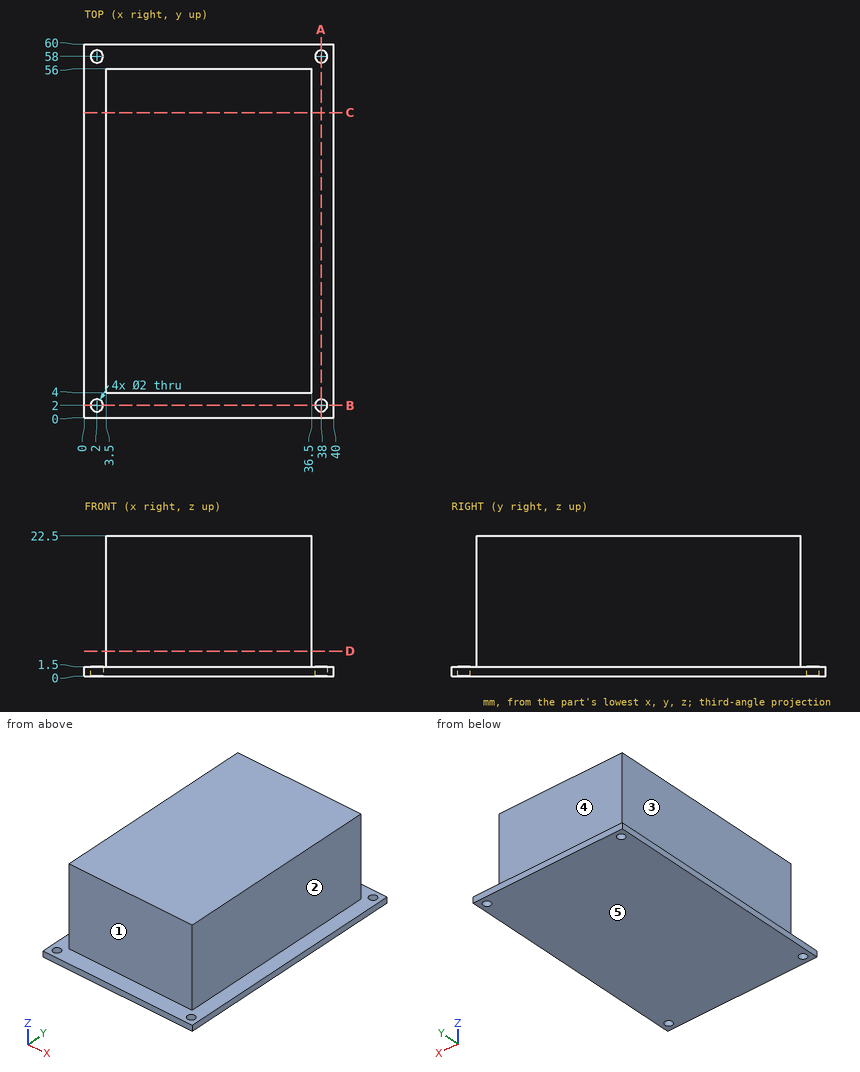
Job drawing, mm, ordinate dimensions from the low corner. One solid piece. A direction names the side the tool comes from. Give positions to 0.01 mm unless a question says otherwise; leave off trailing zeros. Loops run counter-clockwise (first coordinate to the right, second up) from the corner with the lowest first, then second, coordinate; pieces in that order, holes last. Notation, with made-up numbers: M 60,82.5 L 100,82.5 A19 cw 100,112.5 Z; hole C 66.5,44 d6. An arc over 180 degrees is marked long. Put each result on its own line as item: value. Start each with the question number.
1) 3-axis set-ups, long thin cutter, end or side, ignore diameter. For the marked faces 4 and 5: which of +Z, -Z, +X, -X, +Y, -Y reach the whole face in a straight line?
2) Flat gauge pins, fed straight in: pin 1 (6.5 mm diameter, centred on x = 19.5, z = 8, fed in from +Y); pin 2 (1.5 mm diameter, centred on x = 20, z = 7, fed in from -Y); pin 3 (1.8 mm diameter, centred on x = 38, y = 58, fed in from -Z); pin 4 (2.5 mm diameter, centred on x = 38, y = 2, fed in from +Z). Where does each tip first touch, or does it go through?
3) Probe probe 1 along Y at (x, z) = (38, 0.45); probe 2 along X at (y, z) = (58, 1.1); probe 3 along X at (y, z) = (33, 2). List the from-to ranges inside material, lowest first.
4) Saw through at C-C (y = 49). List the corners of the cut face in (x, z), then the cut area to 3 significant figures.
5) Saw through at D-D (z = 4). List the corners of the cut face in (x, y).
6) Saw through at B-B (y = 2). List the corners of the cut face in (x, z), then the cut area to 3 significant figures.
7) Pull direction X, two halves, no side cores. Call the marked faces 1, 2 and 3: +X half, -X half, draft (parallel to the pull), parting line (faces both ways), or undercut.
8) Saw through at A-A (x = 38). List the corners of the cut face in (y, z).
Numbers:
1. face 4: +Z, +X, -X, +Y
1. face 5: -Z, +X, -X, +Y, -Y
2. pin 1: y = 56
2. pin 2: y = 4
2. pin 3: through
2. pin 4: z = 1.5
3. probe 1: 0 to 1, 3 to 57, 59 to 60
3. probe 2: 0 to 1, 3 to 37, 39 to 40
3. probe 3: 3.5 to 36.5
4. outline: M 0,0 L 40,0 L 40,1.5 L 36.5,1.5 L 36.5,22.5 L 3.5,22.5 L 3.5,1.5 L 0,1.5 Z
4. area: 753 mm^2
5. outline: M 3.5,4 L 36.5,4 L 36.5,56 L 3.5,56 Z
6. outline: M 0,0 L 1,0 L 1,1.5 L 0,1.5 Z; M 3,0 L 37,0 L 37,1.5 L 3,1.5 Z; M 39,0 L 40,0 L 40,1.5 L 39,1.5 Z
6. area: 54.0 mm^2
7. face 1: draft
7. face 2: +X half
7. face 3: -X half
8. outline: M 0,0 L 1,0 L 1,1.5 L 0,1.5 Z; M 3,0 L 57,0 L 57,1.5 L 3,1.5 Z; M 59,0 L 60,0 L 60,1.5 L 59,1.5 Z
